Could you check a few things on this model? Use its own coordinates, in mm. A direction names the side the tool comes from. Give positions to 0.01 mm unless a question says otherwise; leave off trailing zeros. Loops run counter-clockwise (first coordinate to the right, second up) from the corner with the lowest first, then second, coordinate; pieces in that order, holes last. Notation, with made-up numbers: (48, 53) - (66, 53) arc R33 cw to (66, 87) - close; hole circle Ø7 at (-25, 0). An arc over 180 degrees is marked (long way). Write each question's results on one line, items separated by ' | '. Start each with the question number.
1) I'm going to push flat-ended pins straight in: pin 1 (6 mm diameter, centred on y = 32, z = 7, fed in from +X); pin 2 (5 mm diameter, centred on x = -3, y = -4, fed in from -Z); pin 3 (2 mm diameter, centred on x = 5.75, y = -9.49, fed in from -Z); pin 4 (1.5 mm diameter, centred on y = -37, z = 7.5, fed in from -X). Where does each tip first touch, or does it pass through?
2) I want a section at A-A, the plane z = 6.75. Write out the boundary of the cut face in (x, y).
3) I want a section at C-C, the plane y = 0. Write out the boundary of the cut face in (x, z).
4) If we mould it in two halves opening along X, with no side actions, what happens to faces 1 (the face through (1, -7, 7.874)), 2 (the face through (-46.03, -14.5, 6.51)), 3 (the face through (1, 10, 13.208))? For each: +X half, -X half, draft (parallel to the pull), parting line (faces both ways), or undercut.
5) If I drill on probe 1 along Y at (x, z) = (0, 3); probe 2 along Y at (x, z) = (-5.75, 3); probe 3 along Y at (x, z) = (-1, 5.75), over which ranges is the centre line in solid material (lowest first)? Write a range as [from, to].
6) On a 3-axis mill with a long thin cutter (end or side, diameter ignored), from which of +Z, -Z, +X, -X, +Y, -Y can I reach the whole of each face in a straight line? I mean faces 4 (the face through (-6.718, -19.472, 6.512)), 5 (the face through (8, 2.5, 2.6)), 6 (the face through (8, 2.5, 10.6)). Say none if no direction works.
7) I want a section at B-B, the plane x = 0. Write out the boundary of the cut face in (y, z), and give its area (3 significant figures).
8) I want a section at D-D, the plane y = -20.99. Write out the boundary of the cut face in (x, z), and give its area (3 significant figures).
from build123d import *

# Parameters (mm, degrees)
SKETCH1_R           = 48.26
BOSS_EXTRUDE1_DEPTH = 13.208
SKETCH2_R           = 8.382
CUT_EXTRUDE1_DEPTH  = 5.334
SKETCH12_R          = 4.25
CUT_EXTRUDE5_DEPTH  = 70.516231659
SKETCH13_R          = 1.8
CUT_EXTRUDE7_DEPTH  = 70.516231659
SKETCH14_R          = 6.858
CUT_EXTRUDE8_DEPTH  = 70.516231659


with BuildPart() as part:
    # Sketch1 → Boss-Extrude1 (new body)
    with BuildSketch(Plane.XY):
        with Locations(Location((0, 0, 0), (0, 0, 180))):
            Circle(SKETCH1_R)
    extrude(amount=BOSS_EXTRUDE1_DEPTH)

    # Sketch2 → Cut-Extrude1 (cut)
    with BuildSketch(Plane.XY.offset(13.208)):
        Circle(SKETCH2_R)
    cut_extrude1 = extrude(amount=-CUT_EXTRUDE1_DEPTH, mode=Mode.SUBTRACT)

    # Sketch12 → Cut-Extrude5 (cut, through all)
    with BuildSketch(Plane(origin=(0, 0, 0), x_dir=(-1, 0, 0), z_dir=(0, 0, -1))):
        with Locations((0, -15.24)):
            Circle(SKETCH12_R)
    extrude(amount=-CUT_EXTRUDE5_DEPTH, mode=Mode.SUBTRACT)

    # Sketch13 → Cut-Extrude7 (cut, through all)
    with BuildSketch(Plane(origin=(0, 0, 0), x_dir=(-1, 0, 0), z_dir=(0, 0, -1))):
        with Locations((5.75, -9.49)):
            Circle(SKETCH13_R)
        with Locations((5.75, -20.99)):
            Circle(SKETCH13_R)
        with Locations((-5.75, -20.99)):
            Circle(SKETCH13_R)
        with Locations((-5.75, -9.49)):
            Circle(SKETCH13_R)
    extrude(amount=-CUT_EXTRUDE7_DEPTH, mode=Mode.SUBTRACT)

    # Mirror1: Cut-Extrude1 across plane
    add(cut_extrude1.mirror(Plane.XY.offset(6.604)), mode=Mode.SUBTRACT)

    # Sketch14 → Cut-Extrude8 (cut, through all)
    with BuildSketch(Plane.XY.offset(13.208)):
        Circle(SKETCH14_R)
    extrude(amount=-CUT_EXTRUDE8_DEPTH, mode=Mode.SUBTRACT)


solid = part.part
Answers:
1) pin 1: stops at x = 38.57 | pin 2: stops at z = 5.33 | pin 3: passes through | pin 4: stops at x = -31.86
2) outline: circle Ø96.52 at (0, 0); hole circle Ø3.6 at (-5.75, -20.99); hole circle Ø3.6 at (-5.75, -9.49); hole circle Ø13.72 at (0, 0); hole circle Ø8.5 at (0, -15.24); hole circle Ø3.6 at (5.75, -20.99); hole circle Ø3.6 at (5.75, -9.49)
3) outline: (-48.26, 0) - (-8.38, 0) - (-8.38, 5.33) - (-6.86, 5.33) - (-6.86, 7.87) - (-8.38, 7.87) - (-8.38, 13.21) - (-48.26, 13.21) - close; (6.86, 5.33) - (8.38, 5.33) - (8.38, 0) - (48.26, 0) - (48.26, 13.21) - (8.38, 13.21) - (8.38, 7.87) - (6.86, 7.87) - close
4) face 1: undercut | face 2: parting line | face 3: draft
5) probe 1: y = [-48.26, -19.49], [-10.99, -8.38], [8.38, 48.26] | probe 2: y = [-47.92, -22.79], [-19.19, -11.29], [-7.69, -6.1], [6.1, 47.92] | probe 3: y = [-48.25, -19.37], [-11.11, -6.78], [6.78, 48.25]
6) face 4: +Z, -Z | face 5: -Z | face 6: +Z
7) outline: (-48.26, 0) - (-19.49, 0) - (-19.49, 13.21) - (-48.26, 13.21) - close; (-10.99, 0) - (-8.38, 0) - (-8.38, 5.33) - (-6.86, 5.33) - (-6.86, 7.87) - (-8.38, 7.87) - (-8.38, 13.21) - (-10.99, 13.21) - close; (6.86, 5.33) - (8.38, 5.33) - (8.38, 0) - (48.26, 0) - (48.26, 13.21) - (8.38, 13.21) - (8.38, 7.87) - (6.86, 7.87) - close | area: 949 mm2
8) outline: (-43.46, 0) - (-7.55, 0) - (-7.55, 13.21) - (-43.46, 13.21) - close; (-3.95, 0) - (3.95, 0) - (3.95, 13.21) - (-3.95, 13.21) - close; (7.55, 0) - (43.46, 0) - (43.46, 13.21) - (7.55, 13.21) - close | area: 1,050 mm2
